For this review, take the finished solid that the model builds, in its own axes (mm). Face numbers are marked on the shaded views. A direction names the side the tool comes from. Give positions to 0.01 mm unless a question says otherwise; leave off trailing zeros. Loops run counter-clockwise (first coordinate to the right, second up) from the corner with the lowest first, then second, coordinate; pieces in that order, holes last. Notation, with made-up numbers: M 55,-26 L 70,-26 A20 ccw 70,-2 Z; hole C 4,-20.5 d1. An arc over 180 degrees is marked long. Use CSV: the item, a comma, the result in double quotes. Start each with the question number.
1. Insertion check: P1, Ø1.5, axis at x = 7, y = 3.5, coming from the +Z side; P2, Ø2.5, axis at x = 0, y = 0, coming from the -Z side; P3, Ø1, axis at y = 1.5, z = -6.5, coming from the -X side; P4, Ø2, axis at x = 0, y = 4.5, coming from the -Z side. Each pin has a flat end and moves straight along its axis. Give the tip position at first contact, or say it passes through.
2. The part is to be moulded in two halves that separate along Z. For the marked faces 1, 2 and 3, say which applies: pulls with the +Z half, pulls with the -Z half, needs draft (parallel to the pull), parting line crosses it, or undercut.
3. Take a section at A-A, the plane y = 0. Write out the cut boundary in (x, z), and give its area (3 significant figures).
4. Take a section at B-B, the plane x = 4. Write out the cut boundary in (y, z), and give its area (3 significant figures).
5. Tool access review of the marked faces 4, 5, 6, 7 and 8: name each direction out of +Z, -Z, +X, -X, +Y, -Y from which nothing blocks a thin tool from reaching the whole face with its end or side.
6. To check wall thickness, follow line 1 (X direction, y = 6.5, z = -4); line 2 (Y direction, x = 0, z = -0.75); line 3 (X direction, y = -2, z = -7.5). State the ranges of each line that lie inside material, in increasing order. Write a range as [from, to].
7. Take a section at C-C, the plane z = -3.5. State how many separate pieces and enclosed holes the cut face has, and give its area (3 significant figures).
8. Take a section at D-D, the plane x = 9.5. Write out the cut boundary in (y, z).
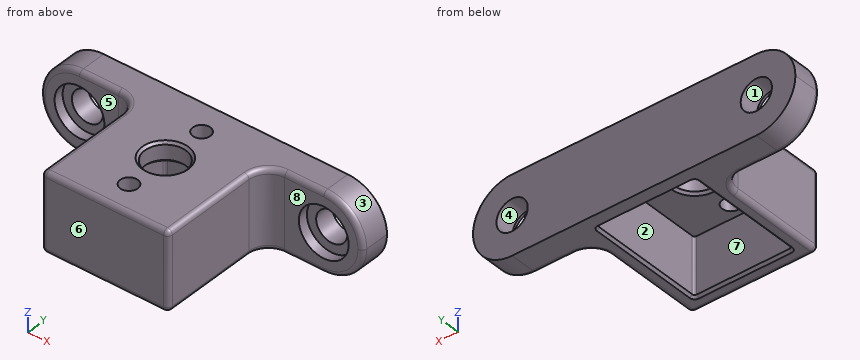
Autodesk Inventor part; units mm, degrees
ref_plane "YZ Plane" through (0, 0, 0) normal (1, 0, 0) x (0, 1, 0)
ref_plane "XZ Plane" through (0, 0, 0) normal (0, 1, 0) x (-1, 0, 0)
ref_plane "XY Plane" through (0, 0, 0) normal (0, 0, 1) x (1, 0, 0)
sketch "Sketch1" plane through (0, 0, 0) normal (0, 1, 0) x (-1, 0, 0)
  point P0 (0, 0)
sketch "Sketch2" plane through (0, 0, 0) normal (0, 0, 1) x (1, 0, 0)
  circle A0 centre (0, -4.5) radius 0.9
  circle A1 centre (0, 4.5) radius 0.9
  circle A2 centre (0, 0) radius 2.0975
  line L0 (6.5, 7.5) -> (-6.5, 7.5)
  line L1 (-6.5, 7.5) -> (-6.5, -7.5)
  line L2 (-6.5, -7.5) -> (6.5, -7.5)
  line L3 (6.5, -7.5) -> (6.5, 7.5)
  dimension "d0" = 1.8
  dimension "d1" = 9
  dimension "d2" = 4.195
  dimension "d3" = 4.5
  dimension "d4" = 13
  dimension "d5" = 15
  dimension "d6" = 7.5
  dimension "d7" = 6.5
extrude "Extrusion1" add sketch "Sketch2" against normal blind 2
sketch "Sketch3" plane through (0, 0, -2) normal (0, 0, -1) x (-1, 0, 0)
  line L0 (6.5, 7.5) -> (-6.5, 7.5)
  line L1 (-6.5, 7.5) -> (-6.5, -7.5)
  line L2 (6.5, -7.5) -> (6.5, 7.5)
  line L3 (-6.5, -7.5) -> (6.5, -7.5)
  line L4 (-5, 6) -> (5, 6)
  line L5 (5, 6) -> (5, -6)
  line L6 (5, -6) -> (-5, -6)
  line L7 (-5, -6) -> (-5, 6)
  point P0 (0, 0)
  dimension "d10" = 1.5
  dimension "d11" = 1.5
  dimension "d12" = 1.5
  dimension "d13" = 1.5
extrude "Extrusion2" add sketch "Sketch3" along normal blind 6
sketch "Sketch4" plane through (-6.5, 7.5, 0) normal (0, 1, 0) x (1, 0, 0)
  line L0 (13, 8) -> (0, 8)
  line L1 (0, 8) -> (-10, 8)
  line L2 (-10, 8) -> (-10, 0)
  line L3 (0, 0) -> (13, 0)
  line L4 (-10, 0) -> (0, 0)
  line L5 (13, 0) -> (23, 0)
  line L6 (23, 0) -> (23, 8)
  line L7 (23, 8) -> (13, 8)
  line L8 (0, 0) -> (0, 8)
  line L9 (13, 0) -> (13, 8)
  circle A0 centre (-6, 4) radius 1.6
  circle A1 centre (19, 4) radius 1.6
  point P0 (6.5, 0)
  point P1 (-10, 4)
  point P2 (-5, 0)
  point P3 (18, 0)
  dimension "d16" = 3.2
  dimension "d17" = 10
  dimension "d22" = 4
  dimension "d23" = 4
extrude "Extrusion3" add sketch "Sketch4" against normal blind 3 contours L7 L6 L5 L9 | L8 L4 L2 L1
fillet "Fillet1" radius 2 2 edges at (-6.5, 4.5, -4) (6.5, 4.5, -4)
fillet "Fillet2" radius 4 4 edges at (-16.5, 6, 0) (-16.5, 6, -8) (16.5, 6, 0) (16.5, 6, -8)
sketch "Sketch5" plane through (-6.5, 4.5, 0) normal (0, -1, 0) x (1, 0, 0)
  circle A0 centre (19, -4) radius 1.6
  circle A1 centre (-6, -4) radius 1.6
  circle A2 centre (19, -4) radius 2.55
  circle A3 centre (-6, -4) radius 2.55
  point P0 (6.5, 0)
  dimension "d24" = 5.1
extrude "Extrusion4" cut sketch "Sketch5" against normal blind 1
fillet "Fillet3" radius 0.5 16 edges at (-6.5, -7.5, -4) (6.5, -7.5, -4) (-10.5002, 4.5, 0) (-15.3286, 4.5, -1.1714) (-16.5, 4.5, -4) (-10.5003, 4.5, -8) (-6.5, -2.5, -8) (-6.5, -2.5, 0) (10.5002, 4.5, 0) (15.3286, 4.5, -1.1714) (16.5, 4.5, -4) (10.5003, 4.5, -8) (6.5, -2.5, -8) (6.5, -2.5, 0) (0, -7.5, 0) (0, -7.5, -8)
fillet "Fillet4" radius 0.25 4 edges at (5, -6, -5) (-5, -6, -5) (5, 6, -5) (-5, 6, -5)
chamfer "Chamfer1" distance 0.25 angle 45 10 edges at (-2.0975, 0, -2) (-2.0975, 0, 0) (0, -6, -8) (4.9268, -5.9268, -8) (5, 0, -8) (4.9268, 5.9268, -8) (0, 6, -8) (-4.9268, 5.9268, -8) (-5, 0, -8) (-4.9268, -5.9268, -8)
properties part number "v2motormount"
Result set:
1,P1,"z = 0"
1,P2,"through"
1,P3,"x = -6.5"
1,P4,"z = -2"
2,face 1,"undercut"
2,face 2,"needs draft"
2,face 3,"pulls with the +Z half"
3,outline,"M -6.5,-7.5 A0.5 ccw -6,-8 L -5.25,-8 L -5,-7.75 L -5,-2 L -2.35,-2 L -2.1,-1.75 L -2.1,-0.25 L -2.35,0 L -6,0 A0.5 ccw -6.5,-0.5 Z; M 2.1,-1.75 L 2.35,-2 L 5,-2 L 5,-7.75 L 5.25,-8 L 6,-8 A0.5 ccw 6.5,-7.5 L 6.5,-0.5 A0.5 ccw 6,0 L 2.35,0 L 2.1,-0.25 Z"
3,area,"35.2 mm2"
4,outline,"M -7.5,-7.5 A0.5 ccw -7,-8 L -6.25,-8 L -6,-7.75 L -6,-2 L 6,-2 L 6,-7.75 L 6.25,-8 L 7.5,-8 L 7.5,0 L -7,0 A0.5 ccw -7.5,-0.5 Z"
4,area,"47.8 mm2"
5,face 4,"+Y, -Y"
5,face 5,"+Z, -Z, -X, -Y"
5,face 6,"+Z, -Z, +X, -X, -Y"
5,face 7,"-Z"
5,face 8,"+Z, -Z, +X, -Y"
6,line 1,"[-16.5, -14.1], [-10.9, 10.9], [14.1, 16.5]"
6,line 2,"[-7.5, -5.4], [-3.6, -2.1], [2.1, 3.6], [5.4, 7.5]"
6,line 3,"[-6.5, -5], [5, 6.5]"
7,separate pieces,"3"
7,enclosed holes,"1"
7,area,"114 mm2"
8,outline,"M 4.5,-7.5 A0.5 ccw 5,-8 L 7.5,-8 L 7.5,0 L 5,0 A0.5 ccw 4.5,-0.5 Z"
